Design review of the part built by this model. Coordinates are the model's own, in mm. A direction names the side the tool comes from. Coordinates: 2 decimals unless noted, no trailing zeros. Loops run counter-clockwise (first coordinate to the right, second up) from the corner with the lowest first, then second, coordinate; pieces in that order, holes last. Notation, with made-up numbers: M 44,-10.75 L 91,-10.75 A7 cw 91,-4.75 Z; hole C -31,48.5 d11. An arc over 180 degrees is marked long. Put each result on its own line as item: value. Start each with the question number.
(1) Take a section at D-D, the plane x = -89.5. Give the boundary of the cut face in (y, z), then the cut area to 3 significant figures.
(2) For probe 1 along X at (y, z) = (152.5, 1); probe 2 along Y at (x, z) = (20, 0.95); probe 3 along Y at (x, z) = (19.5, 0.3), list the stretches that pass through material, from the lowest coordinate up. Write a range as [from, to].
(3) Take a section at A-A, the plane x = 5. Give the boundary of the cut face in (y, z).
(4) Take a section at C-C, the plane z = 2.15. Count the separate pieces of the cut face and the enclosed holes in it, then the cut area to 3 significant figures.
(5) Clearance check with flat-ended pins moving along their axes: pin 1 (1 mm diameter, centred on x = -33.5, z = 2.5, fed in from -Y); pin 2 (5.5 mm diameter, centred on x = 5, y = -15, fed in from -Z); pin 3 (4 mm diameter, centred on x = 20, y = -15, fed in from +Z); pin 4 (2 mm diameter, centred on y = 141.5, z = 1.5, fed in from +X). State where each tip first meets the part, or that it passes through.
(6) Take a section at B-B, the plane y = 172.5. Give the boundary of the cut face in (x, z).
(7) For faces 4 (the cylindrical face through (-89.96, 107.45, 2.03)), 5 (the flat face through (13, 0, 2)), list the 3-axis set-ups (+Z, -Z, +X, -X, +Y, -Y) from which the entire face can be reached by the end or side of a thin tool; tool diameter is ignored.
(8) The part is to be moulded in two halves that separate along Y. For faces 1 (the cylindrical face through (-73.076, 9.799, 1.972)), 2 (the cylindrical face through (-60, 25, 2)), 3 (the cylindrical face through (-99.96, 107.45, 2.03)), say which applies: +Y half, -Y half, draft (parallel to the pull), parting line (faces both ways), or undercut.
```python
from build123d import *

# Parameters (mm, degrees)
EXTRUDE_1_DEPTH     = 4
SKETCH_5_W          = 20
SKETCH_5_H          = 93
EXTRUDE_4_DEPTH     = 4
SKETCH_6_W          = 30
SKETCH_6_H          = 20
EXTRUDE_5_DEPTH     = 4
SKETCH_7_R          = 2.1
CUT_EXTRUDE_2_DEPTH = 5
FILLET_2_R          = 3


with BuildPart() as part:
    # 草图1 → 凸台-拉伸1 (new body)
    with BuildSketch(Plane.XY):
        with BuildLine():
            Line((0, 0), (0, -20))
            ThreePointArc((0, -20), (-73.892658634, 10.607341366), (-104.5, 84.5))
            Line((-104.5, 84.5), (-84.5, 84.5))
            ThreePointArc((-84.5, 84.5), (-59.75052301, 24.74947699), (0, 0))
        make_face()
    extrude(amount=EXTRUDE_1_DEPTH)

    # 草图5 → 凸台-拉伸4 (add)
    with BuildSketch(Plane.XY.offset(4)):
        with Locations((-94.5, 131)):
            Rectangle(SKETCH_5_W, SKETCH_5_H)
    extrude(amount=-EXTRUDE_4_DEPTH)

    # 草图6 → 凸台-拉伸5 (add)
    with BuildSketch(Plane.XY.offset(4)):
        with Locations((15, -10)):
            Rectangle(SKETCH_6_W, SKETCH_6_H)
    extrude(amount=-EXTRUDE_5_DEPTH)

    # 草图7 → 切除-拉伸2 (cut, through all)
    with BuildSketch(Plane.XY.offset(4)):
        with Locations((-99.5, 109.5)):
            Circle(SKETCH_7_R)
        with Locations((-89.5, 109.5)):
            Circle(SKETCH_7_R)
        with Locations((-89.5, 89.5)):
            Circle(SKETCH_7_R)
        with Locations((-99.5, 89.5)):
            Circle(SKETCH_7_R)
        with Locations((-99.5, 152.5)):
            Circle(SKETCH_7_R)
        with Locations((-89.5, 152.5)):
            Circle(SKETCH_7_R)
        with Locations((-89.5, 172.5)):
            Circle(SKETCH_7_R)
        with Locations((-99.5, 172.5)):
            Circle(SKETCH_7_R)
        with Locations((20, -15)):
            Circle(SKETCH_7_R)
        with Locations((20, -5)):
            Circle(SKETCH_7_R)
        with Locations((5, -5)):
            Circle(SKETCH_7_R)
        with Locations((5, -15)):
            Circle(SKETCH_7_R)
    extrude(amount=-CUT_EXTRUDE_2_DEPTH, mode=Mode.SUBTRACT)

    # 圆角2
    fillet_2_edges = [part.edges().sort_by_distance(p)[0] for p in [
        (-104.5, 177.5, 2),
        (-84.5, 177.5, 2),
        (30, 0, 2),
        (30, -20, 2),
    ]]
    fillet(fillet_2_edges, radius=FILLET_2_R)


solid = part.part
```
Computed values:
1. outline: M 30.56,0 L 87.4,0 L 87.4,4 L 30.56,4 Z; M 91.6,0 L 107.4,0 L 107.4,4 L 91.6,4 Z; M 111.6,0 L 150.4,0 L 150.4,4 L 111.6,4 Z; M 154.6,0 L 170.4,0 L 170.4,4 L 154.6,4 Z; M 174.6,0 L 177.5,0 L 177.5,4 L 174.6,4 Z
1. area: 521 mm^2
2. probe 1: x = [-104.5, -101.6], [-97.4, -91.6], [-87.4, -84.5]
2. probe 2: y = [-20, -17.1], [-12.9, -7.1], [-2.9, 0]
2. probe 3: y = [-20, -17.04], [-12.96, -7.04], [-2.96, 0]
3. outline: M -20,0 L -17.1,0 L -17.1,4 L -20,4 Z; M -12.9,0 L -7.1,0 L -7.1,4 L -12.9,4 Z; M -2.9,0 L 0,0 L 0,4 L -2.9,4 Z
4. separate pieces: 1
4. enclosed holes: 12
4. area: 5,250 mm^2
5. pin 1: stops at y = -14.65
5. pin 2: stops at z = 0
5. pin 3: passes through
5. pin 4: stops at x = -84.5
6. outline: M -104.5,0 L -101.6,0 L -101.6,4 L -104.5,4 Z; M -97.4,0 L -91.6,0 L -91.6,4 L -97.4,4 Z; M -87.4,0 L -84.5,0 L -84.5,4 L -87.4,4 Z
7. face 4: +Z, -Z
7. face 5: +Z, -Z, +X, +Y
8. face 1: -Y half
8. face 2: +Y half
8. face 3: undercut
